```python
from build123d import *

# Parameters (mm, degrees)
BOSS_EXTRUDE1_DEPTH = 25.4
SKETCH4_R           = 3.302
BOSS_EXTRUDE2_DEPTH = 25.4
SKETCH6_R           = 1.778
CUT_EXTRUDE1_DEPTH  = 74.551770003


with BuildPart() as part:
    # Sketch3 → Boss-Extrude1 (new body)
    with BuildSketch(Plane.XY):
        with BuildLine():
            Line((42.012655142, -6.604), (30.128190046, -6.604))
            ThreePointArc((30.128190046, -6.604), (15.269190046, -21.463), (30.128190046, -36.322))
            Line((30.128190046, -36.322), (42.012655142, -36.322))
            Line((42.012655142, -36.322), (42.012655142, -52.07))
            Line((42.012655142, -52.07), (0, -52.07))
            Line((0, -52.07), (0, 0))
            Line((0, 0), (42.012655142, 0))
            Line((42.012655142, 0), (42.012655142, -6.604))
        make_face()
    extrude(amount=BOSS_EXTRUDE1_DEPTH)

    # Sketch4 → Boss-Extrude2 (add)
    with BuildSketch(Plane.XY.offset(25.4)):
        with Locations((42.012655142, -3.302)):
            Circle(SKETCH4_R)
        with Locations((42.012655142, -39.624)):
            Circle(SKETCH4_R)
        with Locations((42.012655142, -48.768)):
            Circle(SKETCH4_R)
    extrude(amount=-BOSS_EXTRUDE2_DEPTH)

    # Sketch6 → Cut-Extrude1 (cut, through all)
    with BuildSketch(Plane.XY.offset(25.4)):
        with Locations((42.012655142, -3.302)):
            Circle(SKETCH6_R)
        with Locations((42.012655142, -39.624)):
            Circle(SKETCH6_R)
        with Locations((42.012655142, -48.768)):
            Circle(SKETCH6_R)
    extrude(amount=-CUT_EXTRUDE1_DEPTH, mode=Mode.SUBTRACT)


solid = part.part
```
For this review, take the finished solid that the model builds, in its own axes (mm). A direction names the side the tool comes from. Round coordinates to 2 decimals unless told otherwise and drop trailing zeros. Write each loop counter-clockwise with the first axis right and the second up, starting at its lowest first coordinate (ties: lowest second). Pieces come first, ordered by that corner, then holes. Notation, with made-up numbers: (-7.5, 19) - (1.5, 19) arc R8 cw to (1.5, 28) - close; hole circle Ø5 at (52, 85.25). An arc over 180 degrees is marked (long way). Use CSV: the item, a comma, the result in double quotes.
1) Wall thickness on line 1 along Y through (x, z) = (36, 13.25); line 2 along X through (y, z) = (-3.5, 8.25); line 3 along Y through (x, z) = (22.5, 9.25): over which ranges is each line inside the solid? List them lowest first. Write a range as from..to.
Conclusion:
line 1,"y = -52.07..-36.32, -6.6..0"
line 2,"x = 0..40.25, 43.78..45.31"
line 3,"y = -52.07..-34.21, -8.71..0"
2) Add section C-C on x = 17. Write out the cut boundary in (y, z).
Conclusion:
outline,"(-52.07, 0) - (-28.42, 0) - (-28.42, 25.4) - (-52.07, 25.4) - close; (-14.5, 0) - (0, 0) - (0, 25.4) - (-14.5, 25.4) - close"
3) Add section B-B on z = 11.5. Write out the cut boundary in (x, y).
Conclusion:
outline,"(0, -52.07) - (42.01, -52.07) arc R3.3 ccw to (42.01, -45.47) - (42.01, -42.93) arc R3.3 ccw to (42.01, -36.32) - (30.13, -36.32) arc R14.86 cw to (30.13, -6.6) - (42.01, -6.6) arc R3.3 ccw to (42.01, 0) - (0, 0) - close; hole circle Ø3.56 at (42.01, -48.77); hole circle Ø3.56 at (42.01, -39.62); hole circle Ø3.56 at (42.01, -3.3)"
4) The part is to be moulded in two halves that separate along X. For faces 1 (the cylindrical face through (43.655, -3.983, 12.878)), 2 (the cylindrical face through (45.314, -3.375, 12.878)), 3 (the flat face through (21, 0, 13)), 4 (the cylindrical face through (42.97, -47.27, 12.88)), say which applies: pulls with the +X half, pulls with the -X half, needs draft (parallel to the pull), parting line crosses it, or undercut.
Conclusion:
face 1,"undercut"
face 2,"pulls with the +X half"
face 3,"needs draft"
face 4,"undercut"
5) Clearance check with a flat-ended pin moving along its axis: pin 1 Ø4 at (y, z) = (-16.5, 21.5) entering from +X. State where the tip first meets the part, or that it passes through.
Conclusion:
pin 1,"stops at x = 17"
6) For faces 5 (the flat face through (0, -26, 13)), 6 (the flat face through (36, -6.604, 13)), list the 3-axis set-ups (+Z, -Z, +X, -X, +Y, -Y) from which the entire face can be reached by the end or side of a thin tool; tool diameter is ignored.
Conclusion:
face 5,"+Z, -Z, -X, +Y, -Y"
face 6,"+Z, -Z, +X"
7) Add section D-D on y = -25. Write out the cut boundary in (x, z), and give its area (3 significant figures).
Conclusion:
outline,"(0, 0) - (15.7, 0) - (15.7, 25.4) - (0, 25.4) - close"
area,"399 mm^2"
8) Add section A-A on x = 35.5. Write out the cut boundary in (y, z), and give its area (3 significant figures).
Conclusion:
outline,"(-52.07, 0) - (-36.32, 0) - (-36.32, 25.4) - (-52.07, 25.4) - close; (-6.6, 0) - (0, 0) - (0, 25.4) - (-6.6, 25.4) - close"
area,"568 mm^2"
